from build123d import *

# Parameters (mm, degrees)
REVOLVE_1_ANGLE     = 180
SKETCH_2_W          = 120
SKETCH_2_H          = 124.466444362
CUT_EXTRUDE_1_DEPTH = 51
SKETCH_3_W          = 10
SKETCH_3_H          = 50
SKETCH_4_W          = 4
SKETCH_4_H          = 40
SKETCH_6_W          = 20
SKETCH_6_H          = 4.5
EXTRUDE_1_DEPTH     = 20
EXTRUDE_3_DEPTH     = 30


with BuildPart() as part:
    # 草图1 → 旋转1 (revolve)
    with BuildSketch(Plane(origin=(0, 0, 0), x_dir=(0, 0, -1), z_dir=(1, 0, 0))):
        Polygon((0, 50), (0, 46), (160, 42), (160, 46), align=None)
    revolve(axis=Axis((0, 0, 0), (0, 0, -1)), revolution_arc=REVOLVE_1_ANGLE)

    # 草图2 → 切除-拉伸1 (cut, through all)
    with BuildSketch(Plane(origin=(0, 0, 0), x_dir=(0, 0, -1), z_dir=(1, 0, 0))):
        with Locations((80, -2.118201403)):
            Rectangle(SKETCH_2_W, SKETCH_2_H)
    extrude(amount=CUT_EXTRUDE_1_DEPTH, mode=Mode.SUBTRACT)

    # 草图3 → 放样1 section 0
    with BuildSketch(Plane.XY):
        with Locations((50, 0)):
            Rectangle(SKETCH_3_W, SKETCH_3_H)
    # 草图4 → 放样1 section 1
    with BuildSketch(Plane(origin=(0, 0, -160), x_dir=(-1, 0, 0), z_dir=(0, 0, -1))):
        with Locations((-44, 0)):
            Rectangle(SKETCH_4_W, SKETCH_4_H)
    loft()

    # 草图6 → 凸台-拉伸1 (add)
    with BuildSketch(Plane.ZY):
        with Locations((-10, 47.75)):
            Rectangle(SKETCH_6_W, SKETCH_6_H)
        with Locations((-10, -47.75)):
            Rectangle(SKETCH_6_W, SKETCH_6_H)
        with Locations((-150, -44.25)):
            Rectangle(SKETCH_6_W, SKETCH_6_H)
        with Locations((-150, 44.25)):
            Rectangle(SKETCH_6_W, SKETCH_6_H)
    extrude(amount=EXTRUDE_1_DEPTH)

    # 草图8 → 凸台-拉伸3 (add)
    with BuildSketch(Plane.XY.offset(-140)):
        with BuildLine():
            Line((0, 46), (0, 50))
            ThreePointArc((0, 50), (50, 0), (0, -50))
            Line((0, -50), (0, -46))
            ThreePointArc((0, -46), (46, 0), (0, 46))
        make_face()
    extrude(amount=-EXTRUDE_3_DEPTH)


solid = part.part
Check sheet for the modelled part. Datum: model origin and axes. Units: mm. A direction names the side the tool comes from. Round coordinates to 2 decimals unless told otherwise and drop trailing zeros. Loops run counter-clockwise (first coordinate to the right, second up) from the corner with the lowest first, then second, coordinate; pieces in that order, holes last.
1. Gauge pin test, flat ends, axial feed: pin 1 Ø6 at (x, z) = (46.5, -151.5) entering from +Y; pin 2 Ø22 at (x, z) = (-12.5, -147) entering from -Y; pin 3 Ø0.6 at (y, z) = (46, -14) entering from +X; pin 4 Ø4.5 at (y, z) = (48.5, -158.5) entering from -X. Record the tip position at first contact, or that the pin passes through.
2. Sectioned sample at A-A on x = -13. Record the boundary of the cut face in (y, z).
3. Sectioned sample at B-B on x = 37. Give the number of separate pieces and of enclosed holes in the cut face, and give its area (3 significant figures).
4. Set-up check for faces 1 (the flat face through (-10, -42, -150)), 2 (the flat face through (-10, 46.5, -150)), 3 (the cylindrical face through (45.99, -1.01, -164.93)), 4 (the cylindrical face through (49.988, 1.099, -154.79)): record each of +Z, -Z, +X, -X, +Y, -Y from which the full face is reachable in a straight line by a thin tool's end or side.
5. Mould release check, pull along Y, two halves, no side actions. Record for faces 5 (the flat face through (-10, -46.5, -150)), 6 (the flat face through (-20, -44, -150)), 7 (the conical face through (28.68, 35.64, -10.14)), 8 (the flat face through (-10, -45.5, -10)): released by +Y, released by -Y, zero draft, split by the parting line, or undercut.
6. Scan lines: probe 1 along Z at (x, y) = (40.5, 28); probe 2 along Y at (x, z) = (-13, -11); probe 3 along Y at (x, z) = (38.5, -150). Record each from-to range of solid material in increasing order.
Recorded:
1. pin 1: stops at y = 24.65
1. pin 2: stops at y = -46.5
1. pin 3: stops at x = 19.41
1. pin 4: stops at x = -20
2. outline: (-50, -20) - (-45.5, -20) - (-45.5, 0) - (-50, 0) - close; (-46.5, -160) - (-42, -160) - (-42, -140) - (-46.5, -140) - close; (42, -160) - (46.5, -160) - (46.5, -140) - (42, -140) - close; (45.5, -20) - (50, -20) - (50, 0) - (45.5, 0) - close
3. separate pieces: 4
3. enclosed holes: 0
3. area: 909 mm2
4. face 1: +Z, -Z, -X
4. face 2: -Z, -X, +Y
4. face 3: -Z, -X
4. face 4: -Z, +X
5. face 5: released by -Y
5. face 6: zero draft
5. face 7: undercut
5. face 8: undercut
6. probe 1: z = -170 to -140, -20 to 0
6. probe 2: y = -50 to -45.5, 45.5 to 50
6. probe 3: y = -31.9 to -17.4, 17.4 to 31.9
